Geometry: final body of the model. Coordinates: model frame, mm. A direction names the side the tool comes from. Coordinates: 2 decimals unless noted, no trailing zeros. Write each loop counter-clockwise with the first axis right and the second up, starting at its lowest first coordinate (ties: lowest second). Pieces come first, ordered by that corner, then holes. Notation, with made-up numbers: (52, 54) - (73, 54) arc R11 cw to (73, 72) - close; hole circle Ø10 at (57, -25). An arc over 180 degrees is marked (long way). Put each result on its own line as item: value.
```python
from build123d import *

# Parameters (mm, degrees)
SKETCH1_W           = 101.599999998
SKETCH1_H           = 101.6
SKETCH1_R           = 2.032
SKETCH1_R_2         = 1.778
SKETCH1_W_2         = 7.62
SKETCH1_H_2         = 7.62
BOSS_EXTRUDE1_DEPTH = 5.9944


with BuildPart() as part:
    # Sketch1 → Boss-Extrude1 (new body)
    with BuildSketch(Plane(origin=(0, 0, 0), x_dir=(0, 0, -1), z_dir=(1, 0, 0))):
        Rectangle(SKETCH1_W, SKETCH1_H)
        with Locations(Location((-40.513, 40.513, 0), (0, 0, 180))):
            Circle(SKETCH1_R, mode=Mode.SUBTRACT)
        with Locations(Location((40.513, 40.513, 0), (0, 0, 180))):
            Circle(SKETCH1_R, mode=Mode.SUBTRACT)
        with Locations(Location((40.513, -40.513, 0), (0, 0, 180))):
            Circle(SKETCH1_R, mode=Mode.SUBTRACT)
        with Locations(Location((-40.513, -40.513, 0), (0, 0, 180))):
            Circle(SKETCH1_R, mode=Mode.SUBTRACT)
        with Locations(Location((-13.4747, 13.4747, 0), (0, 0, 180))):
            Circle(SKETCH1_R_2, mode=Mode.SUBTRACT)
        with Locations(Location((-13.4747, -13.4747, 0), (0, 0, 180))):
            Circle(SKETCH1_R_2, mode=Mode.SUBTRACT)
        with Locations(Location((13.4747, -13.4747, 0), (0, 0, 180))):
            Circle(SKETCH1_R_2, mode=Mode.SUBTRACT)
        with Locations(Location((13.4747, 13.4747, 0), (0, 0, 180))):
            Circle(SKETCH1_R_2, mode=Mode.SUBTRACT)
        with Locations((-0.004315818, 0.004315818)):
            Rectangle(SKETCH1_W_2, SKETCH1_H_2, mode=Mode.SUBTRACT)
    extrude(amount=BOSS_EXTRUDE1_DEPTH)


solid = part.part
```
1. Ray query, probe 1 along Z at (x, y) = (0.85, 0.5); probe 2 along Y at (x, z) = (5.7, -14); probe 3 along Y at (x, z) = (4.3, -42). Return the intervals inside material, ascending. Write a range as from..to.
Answer below:
probe 1: z = -50.8..-3.81, 3.81..50.8
probe 2: y = -50.8..-15.17, -11.78..11.78, 15.17..50.8
probe 3: y = -50.8..-41.9, -39.13..39.13, 41.9..50.8
2. Mould query, pull axis Z, two halves, no side actions, for faces 1 (the flat face through (3, 0, -3.806)), 2 (the flat face through (3, -1, 50.8)), 3 (the flat face through (5.994, 1, 12)). Classes: +Z half, -Z half, draft (parallel to the pull), parting line (faces both ways), or undercut.
Answer below:
face 1: undercut
face 2: +Z half
face 3: draft
3. Set-up query: faces 4 (the flat face through (3, 3.814, 0)), 5 (the flat face through (3, -1, -50.8)). Return all of +Z, -Z, +X, -X, +Y, -Y with unobstructed straight access to the full face (end or side cutting, diameter ignored); none if empty.
Answer below:
face 4: +X, -X
face 5: -Z, +X, -X, +Y, -Y
4. Section query B-B (z = -13.5). Return loops of the section in (x, y).
Answer below:
outline: (0, -50.8) - (5.99, -50.8) - (5.99, -15.25) - (0, -15.25) - close; (0, -11.7) - (5.99, -11.7) - (5.99, 11.7) - (0, 11.7) - close; (0, 15.25) - (5.99, 15.25) - (5.99, 50.8) - (0, 50.8) - close
5. Section query A-A (y = 0.5). Return loops of the section in (x, z), then the cut area to 3 significant figures.
Answer below:
outline: (0, -50.8) - (5.99, -50.8) - (5.99, -3.81) - (0, -3.81) - close; (0, 3.81) - (5.99, 3.81) - (5.99, 50.8) - (0, 50.8) - close
area: 563 mm²
6. Pin query (flat end, axial travel): pin 1 Ø4 at (y, z) = (13.47, 13.47) entering from +X. Return the tip coordinate at first contact, or that it passes through.
Answer below:
pin 1: stops at x = 5.99
